For this review, use the dimensioned drawing (mm, ordinates from the lowest corner) and the shaded views. A direction names the side the tool comes from. Coordinates: 2 decimals unless noted, no trailing zeros. Loops run counter-clockwise (first coordinate to the right, second up) from the corner with the lowest first, then second, coordinate; pieces in that order, holes last. Notation, with made-up numbers: (30.5, 47) - (79.5, 47) arc R19 ccw to (79.5, 56) - close; hole circle Ø1 at (74.25, 11.5). An arc over 180 degrees is marked (long way). Answer in a Markdown table with one row per item. Add a question column.
(1) We need section D-D on x = 17.5. Write out the cut boundary in (y, z) (1 decimal).
(2) For line 1 along X through (y, z) = (2.4, 5.08) (1 decimal); line 2 along X through (y, z) = (0.75, 5.08) (1 decimal); line 3 along Y through (x, z) = (24, 8.5) (1 decimal), list the stretches that pass through material, from the lowest coordinate up.
(3) We need section A-A on z = 5.08. Give the number of separate pieces and of enclosed holes in the cut face, plus the area to 3 significant figures.
(4) We need section B-B on y = 12.7. Write out the cut boundary in (x, z) (1 decimal).
(5) For P1, Ø6, axis at y = 8, z = 13.5, coming from the -X side; P2, Ø3.5, axis at x = 45, z = 19.5, coming from the +Y side; P3, Ø1, axis at x = 33, y = 7.5, coming from the -Z side; P4, Ø1, axis at x = 15, z = 9, coming from the +Y side (1 decimal), all flat-tipped, find the tip position at first contact; note any pin that passes through.
(6) We need section C-C on x = 34. Write out the cut boundary in (y, z) (1 decimal).
(7) Machinability: for the marked faces 1, 2 and 3, which of the approach directions +Z, -Z, +X, -X, +Y, -Y give a long, thin tool a straight path to every point of the face, cutting with its end or side? Answer none if there is none.
(8) Mouldability with a two-part tool opening along Y and no side actions: class the marked faces 4, 5, 6 and 7 as +Y half, -Y half, draft (parallel to the pull), parting line (faces both ways), or undercut.
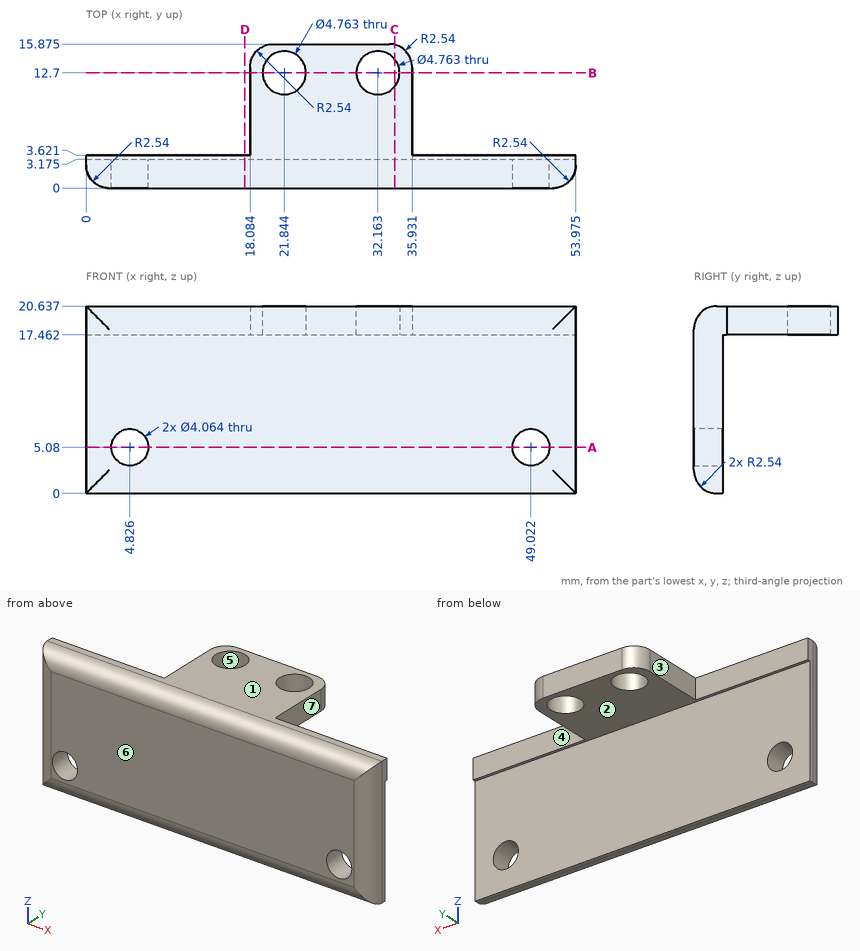
Outcome:
| question | item | result |
|---|---|---|
| 1 | outline | (0, 2.5) arc R2.5 ccw to (2.5, 0) - (3.2, 0) - (3.2, 17.5) - (3.6, 17.5) - (3.6, 20.6) - (2.5, 20.6) arc R2.5 ccw to (0, 18.1) - close |
| 2 | line 1 | 0 to 2.8, 6.9 to 47, 51.1 to 54 |
| 2 | line 2 | 0.7 to 2.8, 6.9 to 47, 51.1 to 53.2 |
| 2 | line 3 | 0 to 3.2 |
| 3 | separate pieces | 3 |
| 3 | enclosed holes | 0 |
| 3 | area | 143 mm² |
| 4 | outline | (18.1, 17.5) - (19.5, 17.5) - (19.5, 20.6) - (18.1, 20.6) - close; (24.2, 17.5) - (29.8, 17.5) - (29.8, 20.6) - (24.2, 20.6) - close; (34.5, 17.5) - (35.9, 17.5) - (35.9, 20.6) - (34.5, 20.6) - close |
| 5 | P1 | through |
| 5 | P2 | y = 3.62 |
| 5 | P3 | z = 17.46 |
| 5 | P4 | y = 3.2 |
| 6 | outline | (0, 2.5) arc R2.5 ccw to (2.5, 0) - (3.2, 0) - (3.2, 17.5) - (11.2, 17.5) - (11.2, 20.6) - (2.5, 20.6) arc R2.5 ccw to (0, 18.1) - close; (14.2, 17.5) - (15.8, 17.5) - (15.8, 20.6) - (14.2, 20.6) - close |
| 7 | face 1 | +Z, +X, -X, +Y, -Y |
| 7 | face 2 | -Z, +X, -X, +Y |
| 7 | face 3 | +Z, -Z, -X, +Y |
| 8 | face 4 | +Y half |
| 8 | face 5 | undercut |
| 8 | face 6 | -Y half |
| 8 | face 7 | draft |
